from build123d import *

# Parameters (mm, degrees)
F1_DEPTH = 150
F2_R     = 5
F3_R     = 2.5
F4_DEPTH = 25


with BuildPart() as f1:
    # F0 (on Front) → F1 (new body)
    with BuildSketch(Plane.XZ):
        Polygon((-47.536419, 35.607496), (-75.006606, -23.30251), (84.993394, -23.30251), (84.993394, 6.69749), (79.993394, 6.69749), (79.993394, -18.30251), (-67.158178, -18.30251), (-43.00488, 33.494404), align=None)
    extrude(amount=F1_DEPTH)

    # F2
    f2_edges = [f1.edges().sort_by_distance(p)[0] for p in [
        (-75.006606, -75, -23.30251),
        (84.993394, -75, -23.30251),
    ]]
    fillet(f2_edges, radius=F2_R)

    # F3 (on face) → F4 (cut)
    with BuildSketch(Plane.YZ.offset(84.993394)):
        with Locations((-115, -3.30251)):
            Circle(F3_R)
        with Locations((-35, -3.30251)):
            Circle(F3_R)
    extrude(amount=-F4_DEPTH, mode=Mode.SUBTRACT)


solid = f1.part
Build history of the part. All positions in model axes, mm. A direction names the side the tool comes from. Coordinates: 2 decimals unless noted, no trailing zeros. Order: outer loops, then holes, each group sorted by start corner. A loop starts at its lowest first (then second) coordinate and runs counter-clockwise, first axis right, second up. Notation, with made-up numbers: (65.5, 63) - (104.5, 63) arc R23 ccw to (104.5, 95) - close; hole circle Ø5 at (19.5, -14.5). An arc over 180 degrees is marked (long way). Write item = value, one per line. Start each with the question number.
1) Saw through at A-A on y = -115. Write the cut outline in (x, z), then the cut area to 3 significant figures.
2) Flat gauge pins, fed straight in: pin 1 Ø6 at (y, z) = (-95.5, 18.5) entering from -X; pin 2 Ø2.5 at (x, y) = (82, -83.5) entering from +Z; pin 3 Ø1.5 at (x, y) = (54, -121) entering from +Z; pin 4 Ø12 at (x, z) = (-45, 14) entering from +Y. Where does each tip first touch, or does it go through?
3) Saw through at D-D on x = 24. Write the cut outline in (y, z).
4) Saw through at C-C on y = -82.5. Write the cut outline in (x, z).
5) Saw through at B-B on z = -12.5. Write the cut outline in (x, y).
6) Wall check: line 1 along Z through (x, y) = (-4.5, -142.5); line 2 along Z through (x, y) = (-53.5, -66); line 3 along Z through (x, y) = (83.7, -35). Give the ranges that are in metal, low to high. Write a range as from..to.
7) Two-plate mould, pull along Y, no slides. Class faces 4 (the face through (-59.444, -73.95, 10.072)), 5 (the face through (0, -150, -20)), 6 (the face through (82.5, -112.6, -2.6)): pulls with the +Y half, pulls with the -Y half, needs draft (parallel to the pull), parting line crosses it, or undercut.
8) 3-axis set-ups, long thin cutter, end or side, ignore diameter. For faces 1 (the face through (82.53, -32.69, -4.26)), 2 (the face through (79.993, -74, -6)), 3 (the face through (83, -74, 6.697)): which of +Z, -Z, +X, -X, +Y, -Y reach the whole face in a straight line?
From the geometry:
q1.outline = (-71.69, -16.19) arc R5 ccw to (-67.16, -23.3) - (79.99, -23.3) arc R5 ccw to (84.99, -18.3) - (84.99, -5.8) - (79.99, -5.8) - (79.99, -18.3) - (-67.16, -18.3) - (-43, 33.49) - (-47.54, 35.61) - close; (79.99, -0.8) - (84.99, -0.8) - (84.99, 6.7) - (79.99, 6.7) - close
q1.area = 1,170 mm^2
q2.pin_1 = -56.91
q2.pin_2 = 6.7
q2.pin_3 = -18.3
q2.pin_4 = through
q3.outline = (-150, -23.3) - (0, -23.3) - (0, -18.3) - (-150, -18.3) - close
q4.outline = (-71.69, -16.19) arc R5 ccw to (-67.16, -23.3) - (79.99, -23.3) arc R5 ccw to (84.99, -18.3) - (84.99, 6.7) - (79.99, 6.7) - (79.99, -18.3) - (-67.16, -18.3) - (-43, 33.49) - (-47.54, 35.61) - close
q5.outline = (-69.97, -150) - (-64.45, -150) - (-64.45, 0) - (-69.97, 0) - close; (79.99, -150) - (84.99, -150) - (84.99, 0) - (79.99, 0) - close
q6.line_1 = -23.3..-18.3
q6.line_2 = -23.3..-18.3, 10.99..22.82
q6.line_3 = -21.66..-5.8, -0.8..6.7
q7.face_4 = needs draft
q7.face_5 = pulls with the -Y half
q7.face_6 = undercut
q8.face_1 = +X
q8.face_2 = +Z, +Y, -Y
q8.face_3 = +Z, +X, +Y, -Y
